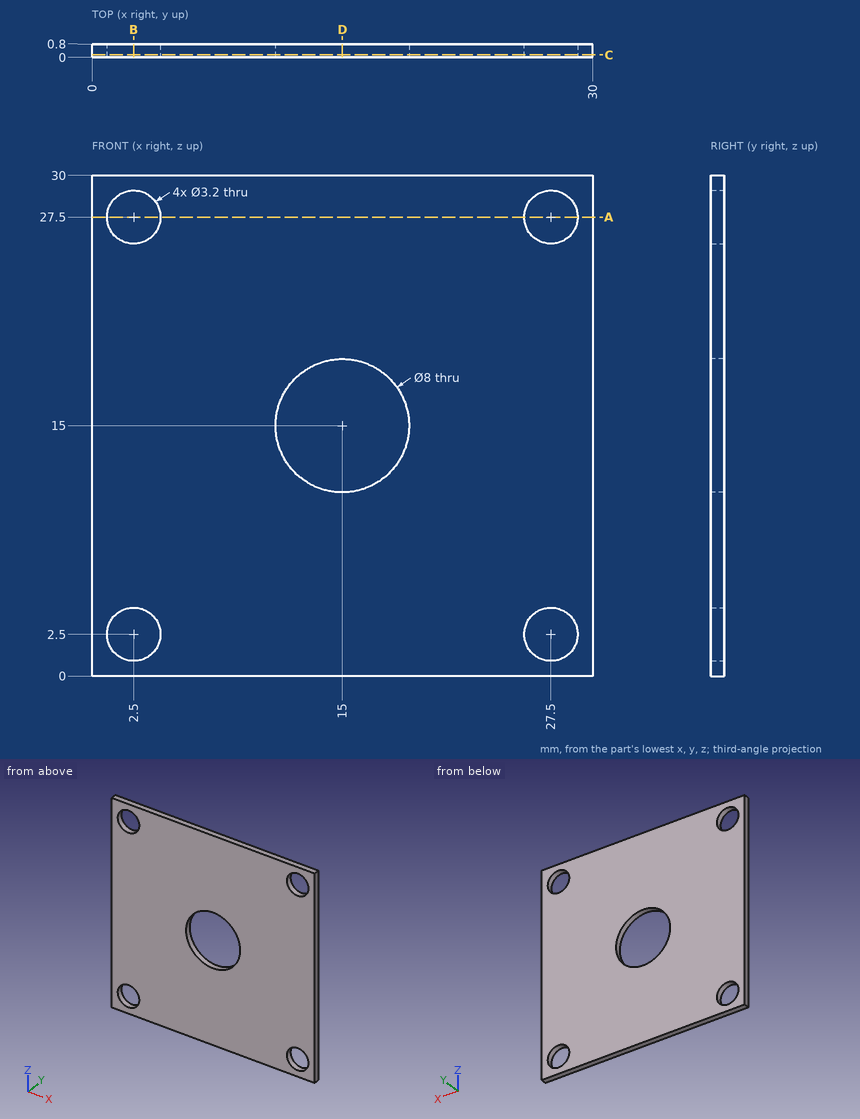
Could you check a few things on this drawing? It's one solid part, dimensions in mm from its lowest x, y, z. Round coordinates to 2 decimals unless told otherwise and drop trailing zeros. Loops run counter-clockwise (first coordinate to the right, second up) from the corner with the lowest first, then second, coordinate; pieces in that order, holes last. Notation, with made-up numbers: (12, 16.5) -> (42, 16.5) arc R32 cw to (42, 44.5) -> close; hole circle Ø10 at (11.5, 46). An arc over 180 degrees is marked (long way). Answer as CSV lines item,"result".
1. If we section it at C-C on y = 0.15: Please give me the cut outline in (x, z).
Final values:
outline,"(0, 0) -> (30, 0) -> (30, 30) -> (0, 30) -> close; hole circle Ø3.2 at (2.5, 2.5); hole circle Ø3.2 at (2.5, 27.5); hole circle Ø8 at (15, 15); hole circle Ø3.2 at (27.5, 2.5); hole circle Ø3.2 at (27.5, 27.5)"
2. For pin 1 (2.5 mm diameter, centred on x = 2.5, z = 27.5, fed in from -Y), with a flat end and sliding along its axis, tell me the tip position at first contact or that it passes through.
Final values:
pin 1,"passes through"
3. If we section it at A-A on z = 27.5: Please give me the cut outline in (x, y).
Final values:
outline,"(0, 0) -> (0.9, 0) -> (0.9, 0.8) -> (0, 0.8) -> close; (4.1, 0) -> (25.9, 0) -> (25.9, 0.8) -> (4.1, 0.8) -> close; (29.1, 0) -> (30, 0) -> (30, 0.8) -> (29.1, 0.8) -> close"
4. If I drill on L1, parallel to Z at x = 27.5, y = 0.5; L2, parallel to Z at x = 3, y = 0.15, over which ranges is the centre line in solid material (lowest first)?
Final values:
L1,"z = 0 to 0.9, 4.1 to 25.9, 29.1 to 30"
L2,"z = 0 to 0.98, 4.02 to 25.98, 29.02 to 30"
5. If we section it at B-B on x = 2.5: Please give me the cut outline in (y, z), plus the area to 3 significant figures.
Final values:
outline,"(0, 0) -> (0.8, 0) -> (0.8, 0.9) -> (0, 0.9) -> close; (0, 4.1) -> (0.8, 4.1) -> (0.8, 25.9) -> (0, 25.9) -> close; (0, 29.1) -> (0.8, 29.1) -> (0.8, 30) -> (0, 30) -> close"
area,"18.9 mm^2"
6. If we section it at D-D on x = 15: Please give me the cut outline in (y, z).
Final values:
outline,"(0, 0) -> (0.8, 0) -> (0.8, 11) -> (0, 11) -> close; (0, 19) -> (0.8, 19) -> (0.8, 30) -> (0, 30) -> close"
